Design review of the part shown in the three views and the two pictorial views. Dimensions are in mm from the part's minimum x, y and z. A direction names the side the tool comes from. Give positions to 0.01 mm unless a question says otherwise; leave off trailing zeros. Loops run counter-clockwise (first coordinate to the right, second up) from the corner with the lowest first, then second, coordinate; pieces in that order, holes last. Notation, with made-up numbers: (32.25, -4.5) -> (66.25, -4.5) arc R25 ccw to (66.25, 31.5) -> close; hole circle Ø2 at (-33, 37.5). An arc over 180 degrees is marked (long way). One line per question, with ' | ' between items. Start each with the question number.
(1) Insertion check: P1, Ø3, axis at x = 2, y = 3.5, coming from the +Z side; P2, Ø3, axis at x = 7, y = 1, coming from the -Z side; P3, Ø1.9, axis at y = 4.5, z = 26.5, coming from the +X side. Each pin has a flat end and moves straight along its axis. Give the tip position at first contact, or say it passes through.
(2) Consider section D-D (y = 5). Write out the cut boundary in (x, z), and give its area (3 significant figures).
(3) Wall thickness on probe 1 along Z at (x, y) = (12, 3.5) (1 decimal); probe 2 along Z at (x, y) = (21, 2.75); probe 3 along X at (y, z) = (1.75, 27.5): over which ranges is each line inside the solid? List them lowest first.
(4) Consider section A-A (z = 26.75). Write out the cut boundary in (x, y).
(5) Tool access review of the marked faces 1, 2 and 3: name each direction out of +Z, -Z, +X, -X, +Y, -Y from which nothing blocks a thin tool from reaching the whole face with its end or side.
(6) Consider section B-B (y = 2.25). Write out the cut boundary in (x, z).
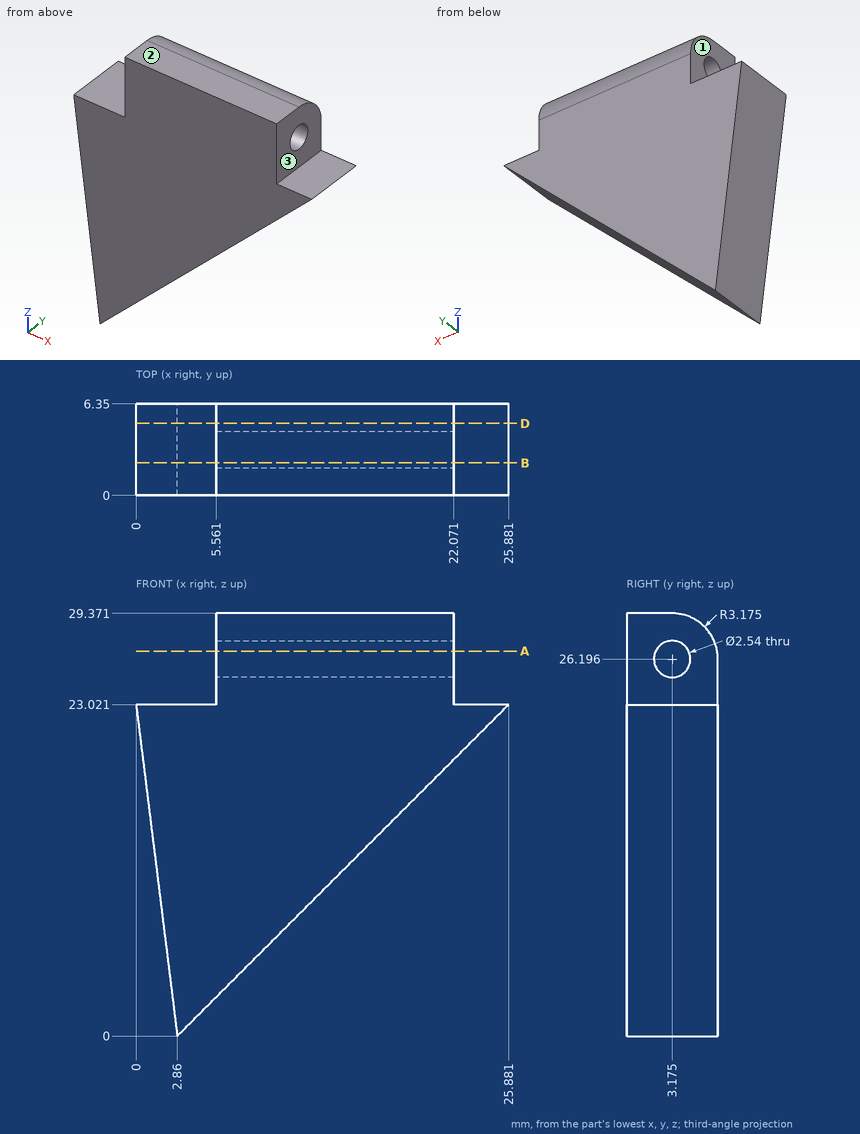
A:
1) P1: stops at z = 23.02 | P2: stops at z = 2.64 | P3: stops at x = 22.07
2) outline: (0, 23.02) -> (2.86, 0) -> (25.88, 23.02) -> (22.07, 23.02) -> (22.07, 28.79) -> (5.56, 28.79) -> (5.56, 23.02) -> close | area: 393 mm^2
3) probe 1: z = 9.1 to 25, 27.4 to 29.4 | probe 2: z = 18.14 to 25, 27.39 to 29.37 | probe 3: x = 5.56 to 22.07
4) outline: (5.56, 0) -> (22.07, 0) -> (22.07, 2.03) -> (5.56, 2.03) -> close; (5.56, 4.32) -> (22.07, 4.32) -> (22.07, 6.3) -> (5.56, 6.3) -> close
5) face 1: +Z, -X, +Y, -Y | face 2: +Z, +X, -X, +Y, -Y | face 3: +Z, +X, +Y, -Y
6) outline: (0, 23.02) -> (2.86, 0) -> (25.88, 23.02) -> (22.07, 23.02) -> (22.07, 25.33) -> (5.56, 25.33) -> (5.56, 23.02) -> close; (5.56, 27.07) -> (22.07, 27.07) -> (22.07, 29.37) -> (5.56, 29.37) -> close
